The listing builds one solid part. Answer for the finished solid, in the listing's coordinates (mm). A direction names the side the tool comes from. Round coordinates to 2 decimals unless told otherwise and drop trailing zeros. Write each loop counter-clockwise with the first axis right and the second up, starting at its lowest first coordinate (ties: lowest second). Pieces come first, ordered by that corner, then holes.
from build123d import *

# Parameters (mm, degrees)
SKETCH1_W           = 50
SKETCH1_H           = 100
SKETCH1_R           = 1.5
SKETCH1_R_2         = 1.35
SKETCH1_W_2         = 30
SKETCH1_H_2         = 30
BOSS_EXTRUDE1_DEPTH = 3.175
CUT_EXTRUDE1_DEPTH  = 6.35


with BuildPart() as part:
    # Sketch1 → Boss-Extrude1 (new body)
    with BuildSketch(Plane(origin=(0, 0, 0), x_dir=(1, 0, 0), z_dir=(0, 1, 0))):
        with Locations((25, -50)):
            Rectangle(SKETCH1_W, SKETCH1_H)
        with Locations(Location((25, -25, 0), (0, 0, 270))):
            Circle(SKETCH1_R, mode=Mode.SUBTRACT)
        with Locations(Location((25, -14.5, 0), (0, 0, 90))):
            Circle(SKETCH1_R_2, mode=Mode.SUBTRACT)
        with Locations(Location((25, -35.5, 0), (0, 0, 270))):
            Circle(SKETCH1_R_2, mode=Mode.SUBTRACT)
        with Locations((25, -65)):
            Rectangle(SKETCH1_W_2, SKETCH1_H_2, mode=Mode.SUBTRACT)
    extrude(amount=BOSS_EXTRUDE1_DEPTH)

    # Sketch2 → Cut-Extrude1 (cut)
    with BuildSketch(Plane(origin=(0, 3.175, 0), x_dir=(1, 0, 0), z_dir=(0, 1, 0))):
        with BuildLine():
            Line((0, 0), (0, -25))
            ThreePointArc((0, -25), (7.32233047, -7.32233047), (25, 0))
            Line((25, 0), (0, 0))
        make_face()
        with BuildLine():
            ThreePointArc((25, 0), (42.67766953, -7.32233047), (50, -25))
            Line((50, -25), (50, 0))
            Line((50, 0), (25, 0))
        make_face()
    extrude(amount=-CUT_EXTRUDE1_DEPTH, mode=Mode.SUBTRACT)


solid = part.part
1. Section B-B on y = 1.3 is taken. Determine the outline of the cut face in (x, z), plus the area to 3 significant figures.
Geometry says:
outline: (0, 25) arc R25 ccw to (50, 25) - (50, 100) - (0, 100) - close; hole (10, 50) - (40, 50) - (40, 80) - (10, 80) - close; hole circle Ø3 at (25, 25); hole circle Ø2.7 at (25, 14.5); hole circle Ø2.7 at (25, 35.5)
area: 3,810 mm2
2. Section D-D on x = 43 is taken. Determine the outline of the cut face in (y, z) (3 decimals).
Geometry says:
outline: (0, 7.651) - (3.175, 7.651) - (3.175, 100) - (0, 100) - close
3. Section A-A on z = 73.5 is taken. Determine the outline of the cut face in (x, y) (3 decimals).
Geometry says:
outline: (0, 0) - (10, 0) - (10, 3.175) - (0, 3.175) - close; (40, 0) - (50, 0) - (50, 3.175) - (40, 3.175) - close
4. Given pin 1 (1.6 mm diameter, centred on x = 29, y = 2, fed in from -Z); pin 2 (2 mm diameter, centred on x = 25, z = 14.5, fed in from -Y), each flat-ended and moving along its own axis, determine where each tip first touches the part or whether it passes through.
Geometry says:
pin 1: stops at z = 0.21
pin 2: passes through
5. For a pull along Z with two mould halves and no side action, classify faces 3 (the face through (25.82, 1.57, 15.57)), 4 (the face through (50, 2, 63)), 5 (the face through (25, 2, 100)) as released by +Z, released by -Z, zero draft, split by the parting line, or undercut.
Geometry says:
face 3: undercut
face 4: zero draft
face 5: released by +Z
6. Section C-C on x = 20.5 is taken. Determine the outline of the cut face in (y, z) (3 decimals).
Geometry says:
outline: (0, 0.408) - (3.175, 0.408) - (3.175, 50) - (0, 50) - close; (0, 80) - (3.175, 80) - (3.175, 100) - (0, 100) - close
7. Straight lines are drawn through the part: line 1 along X through (y, z) = (0.3, 67.5); line 2 along Z through (x, y) = (19, 2.1); line 3 along Z through (x, y) = (10.5, 1.2). For each, find the intervals that lie inside material, in ascending order.
Geometry says:
line 1: x = 0 to 10, 40 to 50
line 2: z = 0.73 to 50, 80 to 100
line 3: z = 4.63 to 50, 80 to 100
8. A tool of negligible diameter and unlimited length cuts with its end or side. For faces 1 (the face through (25, 0, 49)), 2 (the face through (25, 2, 50)), from which of +Z, -Z, +X, -X, +Y, -Y can it reach the whole face along a straight path? Write none if from no direction.
Geometry says:
face 1: +Z, -Z, +X, -X, -Y
face 2: +Y, -Y
